Source: CAD feature listing. Evaluate the final solid. Frame: model axes, mm. A direction names the side the tool comes from. Round coordinates to 2 decimals unless told otherwise and drop trailing zeros. Order: outer loops, then holes, each group sorted by start corner. A loop starts at its lowest first (then second) coordinate and runs counter-clockwise, first axis right, second up. Notation, with made-up numbers: M 40.5,-12.5 L 92.5,-12.5 A9 cw 92.5,-0.5 Z; hole C 30,72 d10. An arc over 180 degrees is marked long. Answer in a Markdown table with one row per item. Add a question column.
```python
from build123d import *

# Parameters (mm, degrees)
CROQUIS1_W              = 95.2
CROQUIS1_H              = 240
SALIENTE_EXTRUIR1_DEPTH = 60
REDONDEO1_R             = 10
VACIADO1_T              = -3


with BuildPart() as part:
    # Croquis1 → Saliente-Extruir1 (new body)
    with BuildSketch(Plane.XY):
        Rectangle(CROQUIS1_W, CROQUIS1_H)
    extrude(amount=SALIENTE_EXTRUIR1_DEPTH)

    # Redondeo1
    redondeo1_edges = [part.edges().sort_by_distance(p)[0] for p in [
        (0, 120, 0),
        (47.6, 0, 0),
        (0, -120, 0),
        (-47.6, 0, 0),
        (-47.6, 120, 30),
        (47.6, 120, 30),
        (47.6, -120, 30),
        (-47.6, -120, 30),
    ]]
    fillet(redondeo1_edges, radius=REDONDEO1_R)

    # Vaciado1
    vaciado1_openings = [part.faces().sort_by_distance(p)[0] for p in [
        (0, 0, 60),
    ]]
    offset(amount=VACIADO1_T, openings=vaciado1_openings, kind=Kind.INTERSECTION)


solid = part.part
```
(1) Cut plane A-A (x = -19). Return loops of the section in (y, z).
(2) Line query: line 1 (Y direction, x = 24.5, z = 52); line 2 (X direction, y = -73, z = 20); line 3 (Z direction, x = 11, y = 44). Output: solid intervals per line, ascending. Write a range as from..to.
(3) Draft query along X for faces 3 (the face through (-44.75, 1.54, 3.01)), 4 (the face through (-1, 120, 35)), 5 (the face through (42.6, 114.9, 35.4)). Return one class per face: +X half, -X half, draft (parallel to the pull), parting line (faces both ways), or undercut.
(4) Pin query (flat end, axial travel): pin 1 (22.5 mm diameter, centred on x = 4.5, y = -27, fed in from +Z). Return the tip coordinate at first contact, or that it passes through.
(5) Cut plane B-B (z = 34). Return loops of the section in (x, y), and give its area (3 significant figures).
(6) Cut plane D-D (z = 7). Return loops of the section in (x, y), and give its area (3 significant figures).
(7) Cut plane C-C (y = 80.5). Return loops of the section in (x, z).
(8) Access query for faces 1 (the face through (44.75, 116.99, 35.35)), 2 (the face through (-42.6, 1.5, 5.1)). Directions: +Z, -Z, +X, -X, +Y, -Y. A direction counts if a zero-diameter tool reaches every point of the face in a straight line with its end or side. Return the directions, or none.
Answer list:
| question | item | result |
|---|---|---|
| 1 | outline | M -120,10 A10 ccw -110,0 L 110,0 A10 ccw 120,10 L 120,60 L 117,60 L 117,10 A7 cw 110,3 L -110,3 A7 cw -117,10 L -117,60 L -120,60 Z |
| 2 | line 1 | -120..-117, 117..120 |
| 2 | line 2 | -47.6..-44.6, 44.6..47.6 |
| 2 | line 3 | 0..3 |
| 3 | face 3 | -X half |
| 3 | face 4 | draft |
| 3 | face 5 | undercut |
| 4 | pin 1 | z = 3 |
| 5 | outline | M -47.6,-110 A10 ccw -37.6,-120 L 37.6,-120 A10 ccw 47.6,-110 L 47.6,110 A10 ccw 37.6,120 L -37.6,120 A10 ccw -47.6,110 Z; hole M -44.6,-110 A7 ccw -37.6,-117 L 37.6,-117 A7 ccw 44.6,-110 L 44.6,110 A7 ccw 37.6,117 L -37.6,117 A7 ccw -44.6,110 Z |
| 5 | area | 1,930 mm² |
| 6 | outline | M -47.14,-110 A9.54 ccw -37.6,-119.54 L 37.6,-119.54 A9.54 ccw 47.14,-110 L 47.14,110 A9.54 ccw 37.6,119.54 L -37.6,119.54 A9.54 ccw -47.14,110 Z; hole M -43.92,-110 A6.32 ccw -37.6,-116.32 L 37.6,-116.32 A6.32 ccw 43.92,-110 L 43.92,110 A6.32 ccw 37.6,116.32 L -37.6,116.32 A6.32 ccw -43.92,110 Z |
| 6 | area | 2,060 mm² |
| 7 | outline | M -47.6,10 A10 ccw -37.6,0 L 37.6,0 A10 ccw 47.6,10 L 47.6,60 L 44.6,60 L 44.6,10 A7 cw 37.6,3 L -37.6,3 A7 cw -44.6,10 L -44.6,60 L -47.6,60 Z |
| 8 | face 1 | +Z, -Z, +X, +Y |
| 8 | face 2 | +Z |
